Autodesk Inventor part; units mm, degrees
ref_plane "YZ Plane" through (0, 0, 0) normal (1, 0, 0) x (0, 1, 0)
ref_plane "XZ Plane" through (0, 0, 0) normal (0, 1, 0) x (-1, 0, 0)
ref_plane "XY Plane" through (0, 0, 0) normal (0, 0, 1) x (1, 0, 0)
sketch "スケッチ1" plane through (0, 0, 0) normal (0, 0, 1) x (1, 0, 0)
  point P0 (0, 0)
sketch "スケッチ2" plane through (0, 0, 0) normal (0, 0, 1) x (1, 0, 0)
  line L0 (0, 0) -> (110, 0)
  line L1 (110, 0) -> (110, -25)
  line L2 (110, -25) -> (0, -25)
  line L3 (0, -25) -> (0, 0)
  ellipse E0 centre (55, -25) end of major axis (110, -25) minor radius 11.2287
  line L4 (0, -25) -> (13.9449, 134.3912)
  line L5 (13.9449, 134.3912) -> (48.8117, 131.3407)
  line L6 (48.8117, 131.3407) -> (34.8668, -28.0505)
  line L7 (34.8668, -28.0505) -> (0, -25)
  circle A0 centre (29.6352, 112.942) radius 14.8
  circle A1 centre (29.6352, 112.942) radius 25
  point P0 (0.0351, -24.599)
  point P1 (36.056, -14.4584)
  point P2 (37.3209, 0)
  dimension "d0" = 110
  dimension "d1" = 25
  dimension "d2" = 35
  dimension "d4" = 160
  dimension "d5" = 5
  dimension "d6" = 29.6
  dimension "d7" = 17.5
  dimension "d18" = 20
  dimension "d23" = 50
extrude "押し出し1" add sketch "スケッチ2" along normal blind 15 contours L4 A1 L6 L0 | L0 L6 E0 L4 | L4 A1 L5 L6 | L4 L5 A1 | A1 L5 L6
extrude "押し出し2" add sketch "スケッチ2" along normal blind 25 contours L4 E0 L6 L2 | L7 L6 L2 E0 | E0 L4 | L2 L6 L7 | L0 L1 E0 L6 | L6 E0 L2
fillet "フィレット1" radius 3 2 edges at (37.3209, 0, 20) (37.3209, 0, 7.5)
fillet "フィレット2" radius 25 1 edges at (110, 0, 12.5)
fillet "フィレット3" radius 15 2 edges at (48.8117, 131.3407, 7.5) (13.9449, 134.3912, 7.5)
fillet "フィレット4" radius 15 1 edges at (36.056, -14.4584, 20)
sketch "スケッチ3" plane through (0, 0, 25) normal (0, 0, 1) x (1, 0, 0)
  line L0 (43.9254, -10.4065) -> (55.2208, -10.4065) construction
  line L1 (55.2208, -10.4065) -> (55.2208, -14.2029) construction
  line L2 (55.2208, -14.2029) -> (43.9254, -14.2029) construction
  line L3 (43.9254, -14.2029) -> (43.9254, -10.4065) construction
  spline S0 degree 2 poles (52.5705, -18.2931) (52.5705, -20.5005) (50.4311, -23.1942) (48.8168, -23.1942) knots 0 0 0 1 2 2 2
  spline S1 degree 2 poles (48.8168, -23.1942) (48.0875, -23.1942) (47.047, -22.8344) (46.5413, -22.5232) knots 0 0 0 1 2 2 2
  line L4 (46.5413, -22.5232) -> (46.444, -22.9414)
  line L5 (46.444, -22.9414) -> (45.0243, -22.9414)
  line L6 (45.0243, -22.9414) -> (45.0243, -10.4065)
  line L7 (45.0243, -10.4065) -> (46.5413, -10.4065)
  line L8 (46.5413, -10.4065) -> (46.5413, -14.8798)
  spline S2 degree 2 poles (46.5413, -14.8798) (47.115, -14.3644) (48.4473, -13.6837) (49.2933, -13.6837) knots 0 0 0 1 2 2 2
  spline S3 degree 2 poles (49.2933, -13.6837) (50.8201, -13.6837) (52.5705, -16.1245) (52.5705, -18.2931) knots 0 0 0 1 2 2 2
  spline S4 degree 2 poles (51.0048, -18.4098) (51.0048, -16.7955) (50.0226, -15.1229) (48.9335, -15.1229) knots 0 0 0 1 2 2 2
  spline S5 degree 2 poles (48.9335, -15.1229) (48.3209, -15.1229) (47.0567, -15.7064) (46.5413, -16.1537) knots 0 0 0 1 2 2 2
  line L9 (46.5413, -16.1537) -> (46.5413, -21.3174)
  spline S6 degree 2 poles (46.5413, -21.3174) (47.115, -21.5994) (48, -21.8328) (48.5251, -21.8328) knots 0 0 0 1 2 2 2
  spline S7 degree 2 poles (48.5251, -21.8328) (49.6823, -21.8328) (51.0048, -20.1893) (51.0048, -18.4098) knots 0 0 0 1 2 2 2
  spline S8 degree 2 poles (61.692, -18.2931) (61.692, -20.5005) (59.5526, -23.1942) (57.9384, -23.1942) knots 0 0 0 1 2 2 2
  spline S9 degree 2 poles (57.9384, -23.1942) (57.209, -23.1942) (56.1685, -22.8344) (55.6628, -22.5232) knots 0 0 0 1 2 2 2
  line L10 (55.6628, -22.5232) -> (55.5656, -22.9414)
  line L11 (55.5656, -22.9414) -> (54.1458, -22.9414)
  line L12 (54.1458, -22.9414) -> (54.1458, -10.4065)
  line L13 (54.1458, -10.4065) -> (55.6628, -10.4065)
  line L14 (55.6628, -10.4065) -> (55.6628, -14.8798)
  spline S10 degree 2 poles (55.6628, -14.8798) (56.2366, -14.3644) (57.5688, -13.6837) (58.4149, -13.6837) knots 0 0 0 1 2 2 2
  spline S11 degree 2 poles (58.4149, -13.6837) (59.9416, -13.6837) (61.692, -16.1245) (61.692, -18.2931) knots 0 0 0 1 2 2 2
  spline S12 degree 2 poles (60.1264, -18.4098) (60.1264, -16.7955) (59.1442, -15.1229) (58.0551, -15.1229) knots 0 0 0 1 2 2 2
  spline S13 degree 2 poles (58.0551, -15.1229) (57.4424, -15.1229) (56.1782, -15.7064) (55.6628, -16.1537) knots 0 0 0 1 2 2 2
  line L15 (55.6628, -16.1537) -> (55.6628, -21.3174)
  spline S14 degree 2 poles (55.6628, -21.3174) (56.2366, -21.5994) (57.1215, -21.8328) (57.6466, -21.8328) knots 0 0 0 1 2 2 2
  spline S15 degree 2 poles (57.6466, -21.8328) (58.8038, -21.8328) (60.1264, -20.1893) (60.1264, -18.4098) knots 0 0 0 1 2 2 2
  line L16 (71.2998, -25.353) -> (62.0421, -25.353)
  line L17 (62.0421, -25.353) -> (62.0421, -24.3125)
  line L18 (62.0421, -24.3125) -> (71.2998, -24.3125)
  line L19 (71.2998, -24.3125) -> (71.2998, -25.353)
  line L20 (79.7309, -22.9414) -> (77.7374, -22.9414)
  line L21 (77.7374, -22.9414) -> (74.3922, -18.5945)
  line L22 (74.3922, -18.5945) -> (73.7893, -19.178)
  line L23 (73.7893, -19.178) -> (73.7893, -22.9414)
  line L24 (73.7893, -22.9414) -> (72.2722, -22.9414)
  line L25 (72.2722, -22.9414) -> (72.2722, -10.4065)
  line L26 (72.2722, -10.4065) -> (73.7893, -10.4065)
  line L27 (73.7893, -10.4065) -> (73.7893, -17.7388)
  line L28 (73.7893, -17.7388) -> (77.3484, -13.9365)
  line L29 (77.3484, -13.9365) -> (79.235, -13.9365)
  line L30 (79.235, -13.9365) -> (75.5397, -17.6999)
  line L31 (75.5397, -17.6999) -> (79.7309, -22.9414)
  line L32 (87.0632, -22.9414) -> (81.209, -22.9414)
  line L33 (81.209, -22.9414) -> (81.209, -21.7161)
  line L34 (81.209, -21.7161) -> (83.3873, -21.7161)
  line L35 (83.3873, -21.7161) -> (83.3873, -13.674)
  line L36 (83.3873, -13.674) -> (81.209, -13.674)
  line L37 (81.209, -13.674) -> (81.209, -12.5751)
  spline S16 degree 2 poles (81.209, -12.5751) (82.444, -12.5751) (83.611, -11.8749) (83.6888, -10.9025) knots 0 0 0 1 2 2 2
  line L38 (83.6888, -10.9025) -> (84.9335, -10.9025)
  line L39 (84.9335, -10.9025) -> (84.9335, -21.7161)
  line L40 (84.9335, -21.7161) -> (87.0632, -21.7161)
  line L41 (87.0632, -21.7161) -> (87.0632, -22.9414)
  point P0 (0, 0)
extrude "押し出し3" cut sketch "スケッチ3" against normal blind 1.2
sketch "スケッチ4" plane through (0, 0, 25) normal (0, 0, 1) x (1, 0, 0)
  circle A0 centre (54.913, -30) radius 3.4
  line L0 (85, 0) -> (40.0699, 0)
  point P0 (0, 0)
  dimension "d19" = 6.8
  dimension "d22" = 30
extrude "押し出し4" cut sketch "スケッチ4" against normal blind 40
extrude "押し出し5" add sketch "スケッチ2" along normal blind 15 contours A1 L4 | L4 A1 L5 L6 | L6 A1 | A1 L5
fillet "フィレット5" radius 15 2 edges at (45.5126, 93.6312, 7.5) (10.6458, 96.6816, 7.5)
equation "\"d7\" = 0.5 * d2"
properties part number "passive_walking_robot1"
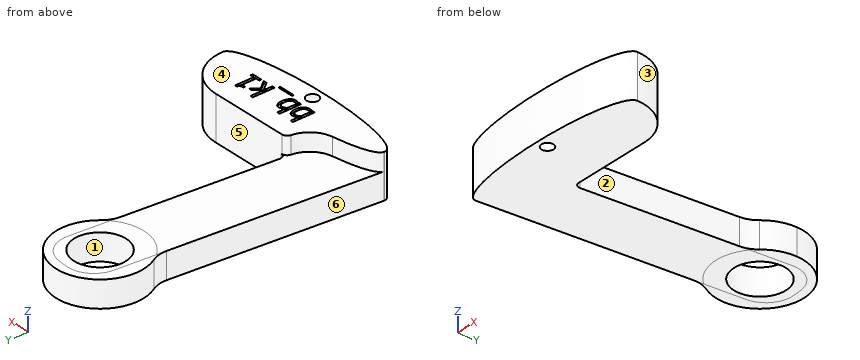
The listing builds one solid part. Answer for the finished solid, in the listing's coordinates (mm). Face numbers are marked on the shaded views. A direction names the side the tool comes from. Coordinates: 2 decimals unless noted, no trailing zeros. Write each loop counter-clockwise with the first axis right and the second up, starting at its lowest first coordinate (ties: lowest second). Pieces come first, ordered by that corner, then holes. Notation, with made-up numbers: M -22,-28.75 L 3,-28.75 A4 ccw 3,-24.75 Z; hole C 83,73.25 d9. An arc over 180 degrees is marked long. Use a Markdown table: item, result. Add a question column.
1. Section C-C (z = 11.5) is taken. Count the separate pieces of the cut face and the enclosed holes in it, plus the area to 3 significant figures.
2. For a pull along Y with two mould halves and no side action, classify the marked faces 3, 4, 5 and 6 as +Y half, -Y half, draft (parallel to the pull), parting line (faces both ways), or undercut.
3. Section D-D (y = 70) is taken. Give the vertices of the cut face in (x, z), plus the area to 3 significant figures.
4. Straight lines are drawn through the part: line 1 along Z through (x, y) = (5, 3.5); line 2 along X through (y, z) = (126, 1); line 3 along Y through (x, z) = (19, 3.75). For each, find the intervals that lie inside material, in ascending order. Write a range as [from, to].
5. Section A-A (y = 126) is taken. Give the vertices of the cut face in (x, z).
6. Section B-B (y = 102) is taken. Give the vertices of the cut face in (x, z).
7. Which of the six approach directions +Z, -Z, +X, -X, +Y, -Y give full straight-line access (tool end or side, diameter ignored) to the marked faces 1 and 2?
8. Given P1, Ø1.5, axis at y = 102, z = 15.5, coming from the -X side; P2, Ø1, axis at y = -19.5, z = 24, coming from the -X side; P3, Ø8, axis at x = 76.5, y = -16, coming from the +Z side; P4, Ø1, axis at x = 54.5, z = 24.5, coming from the +Y side, each flat-ended and moving along its own axis, determine where each tip first touches the part or whether it passes through.
Data:
| question | item | result |
|---|---|---|
| 1 | separate pieces | 1 |
| 1 | enclosed holes | 2 |
| 1 | area | 7,980 mm2 |
| 2 | face 3 | +Y half |
| 2 | face 4 | draft |
| 2 | face 5 | undercut |
| 2 | face 6 | undercut |
| 3 | outline | M 8.31,0 L 43.45,0 L 43.45,15 L 8.31,15 Z |
| 3 | area | 527 mm2 |
| 4 | line 1 | z = [0, 15] |
| 4 | line 2 | x = [8.32, 22.67], [36.6, 50.95] |
| 4 | line 3 | y = [-33.49, 102.65], [123.23, 135.57] |
| 5 | outline | M 8.32,0 L 22.67,0 L 22.67,15 L 8.32,15 Z; M 36.6,0 L 50.95,0 L 50.95,15 L 36.6,15 Z |
| 6 | outline | M 7.16,0 L 19.67,0 L 19.67,15 L 7.16,15 Z; M 39.6,0 L 52.11,0 L 52.11,15 L 39.6,15 Z |
| 7 | face 1 | +Z, -Z |
| 7 | face 2 | +Z, -Z, +X |
| 8 | P1 | stops at x = 6.89 |
| 8 | P2 | stops at x = 5.75 |
| 8 | P3 | stops at z = 25 |
| 8 | P4 | stops at y = 0 |
